```python
from build123d import *

# Parameters (mm, degrees)
F0_R     = 4.25
F1_DEPTH = 55
F2_R     = 4.25
F2_R_2   = 0.35
F3_DEPTH = 3
F4_R     = 4.25
F5_DEPTH = 3
F7_DEPTH = 25


with BuildPart() as f1:
    # F0 (on Top) → F1 (new body)
    with BuildSketch(Plane.XY):
        Circle(F0_R)
        with BuildLine():
            ThreePointArc((0.4014783638, -0.4458868953), (0, -0.6), (-0.4014783638, -0.4458868953))
            Line((-0.4014783638, -0.4458868953), (-1.7825704497, -3.1564327321))
            ThreePointArc((-1.7825704497, -3.1564327321), (-2.1167558909, -2.9427826114), (-2.4255984481, -2.6938999924))
            ThreePointArc((-2.4255984481, -2.6938999924), (-3.1393420887, -1.8125), (-3.5457850527, -0.7536798792))
            ThreePointArc((-3.5457850527, -0.7536798792), (-3.6069024448, -0.3617730694), (-3.6248361561, 0.0344650726))
            Line((-3.6248361561, 0.0344650726), (-0.5868885604, -0.1247470145))
            ThreePointArc((-0.5868885604, -0.1247470145), (-0.5196152423, 0.3), (-0.1854101966, 0.5706339098))
            Line((-0.1854101966, 0.5706339098), (-1.8422657065, 3.1219676595))
            ThreePointArc((-1.8422657065, 3.1219676595), (0, 3.625), (1.8422657065, 3.1219676595))
            Line((1.8422657065, 3.1219676595), (0.1854101966, 0.5706339098))
            ThreePointArc((0.1854101966, 0.5706339098), (0.5196152423, 0.3), (0.5868885604, -0.1247470145))
            Line((0.5868885604, -0.1247470145), (3.6248361561, 0.0344650726))
            ThreePointArc((3.6248361561, 0.0344650726), (3.1393420887, -1.8125), (1.7825704497, -3.1564327321))
            Line((1.7825704497, -3.1564327321), (0.4014783638, -0.4458868953))
        make_face(mode=Mode.SUBTRACT)
    extrude(amount=F1_DEPTH)

    # F2 (on face) → F3 (join)
    with BuildSketch(Plane.XY.offset(55)):
        Circle(F2_R)
        Circle(F2_R_2, mode=Mode.SUBTRACT)
    extrude(amount=F3_DEPTH)

    # F4 (on face) → F5 (join)
    with BuildSketch(Plane.XY.offset(58)):
        Circle(F4_R)
    extrude(amount=F5_DEPTH)

    # F6 (on face) → F7 (join)
    with BuildSketch(Plane.XY.offset(61)):
        with BuildLine():
            ThreePointArc((-2.843805077, -3.1583655083), (-3.6806079661, -2.125), (-4.1571273031, -0.883624686))
            Line((-4.1571273031, -0.883624686), (-5.4765591727, -1.1640785875))
            ThreePointArc((-5.4765591727, -1.1640785875), (-4.8487972217, -2.7994543812), (-3.7464012151, -4.1608000751))
            Line((-3.7464012151, -4.1608000751), (-2.843805077, -3.1583655083))
        make_face()
        with BuildLine():
            ThreePointArc((-1.3133222261, 4.0419901943), (0, 4.25), (1.3133222261, 4.0419901943))
            Line((1.3133222261, 4.0419901943), (1.7301579575, 5.3248786626))
            ThreePointArc((1.7301579575, 5.3248786626), (0, 5.5989087624), (-1.7301579575, 5.3248786626))
            Line((-1.7301579575, 5.3248786626), (-1.3133222261, 4.0419901943))
        make_face()
        with BuildLine():
            ThreePointArc((4.1571273031, -0.883624686), (3.6806079661, -2.125), (2.843805077, -3.1583655083))
            Line((2.843805077, -3.1583655083), (3.7464012151, -4.1608000751))
            ThreePointArc((3.7464012151, -4.1608000751), (4.8487972217, -2.7994543812), (5.4765591727, -1.1640785875))
            Line((5.4765591727, -1.1640785875), (4.1571273031, -0.883624686))
        make_face()
    extrude(amount=-F7_DEPTH)


solid = f1.part
```
Read the model definition and answer for the solid it produces. Units are mm, in the model's axes. A direction names the side the tool comes from. Coordinates: 2 decimals unless noted, no trailing zeros. Loops run counter-clockwise (first coordinate to the right, second up) from the corner with the lowest first, then second, coordinate; pieces in that order, holes last.
(1) The part is cut by section A-A (z = 14.5). Determine the outline of the cut face in (x, y) (3 decimals).
Solution:
outline: circle Ø8.5 at (0, 0); hole (-3.625, 0.034) arc R3.625 ccw to (-1.783, -3.156) - (-0.401, -0.446) arc R0.6 ccw to (0.401, -0.446) - (1.783, -3.156) arc R3.625 ccw to (3.625, 0.034) - (0.587, -0.125) arc R0.6 ccw to (0.185, 0.571) - (1.842, 3.122) arc R3.625 ccw to (-1.842, 3.122) - (-0.185, 0.571) arc R0.6 ccw to (-0.587, -0.125) - close
(2) The part is cut by section B-B (z = 39). Determine the outline of the cut face in (x, y) (3 decimals).
Solution:
outline: (-5.477, -1.164) arc R5.599 ccw to (-3.746, -4.161) - (-2.844, -3.158) arc R4.25 ccw to (2.844, -3.158) - (3.746, -4.161) arc R5.599 ccw to (5.477, -1.164) - (4.157, -0.884) arc R4.25 ccw to (1.313, 4.042) - (1.73, 5.325) arc R5.599 ccw to (-1.73, 5.325) - (-1.313, 4.042) arc R4.25 ccw to (-4.157, -0.884) - close; hole (-3.625, 0.034) arc R3.625 ccw to (-1.783, -3.156) - (-0.401, -0.446) arc R0.6 ccw to (0.401, -0.446) - (1.783, -3.156) arc R3.625 ccw to (3.625, 0.034) - (0.587, -0.125) arc R0.6 ccw to (0.185, 0.571) - (1.842, 3.122) arc R3.625 ccw to (-1.842, 3.122) - (-0.185, 0.571) arc R0.6 ccw to (-0.587, -0.125) - close
(3) The mould has two halves that part along Y. Classify faces 4 (the face through (-4, -2, 36)), 5 (the face through (3.289, -3.653, 48.675)), 6 (the face through (-1.002, 1.828, 27.115)): released by +Y, released by -Y, zero draft, split by the parting line, or undercut.
Solution:
face 4: zero draft
face 5: released by -Y
face 6: undercut
(4) Consider line 1 along Y through (x, z) = (0, 56.3); line 2 along X through (y, z) = (-3.25, 38); line 3 along Y through (x, z) = (-1.5, 33). Determine where each line is inside the solid, lowest interval first.
Solution:
line 1: y = -4.25 to -0.35, 0.35 to 5.6
line 2: x = -4.56 to -2.93, -2.74 to 2.74, 2.93 to 4.56
line 3: y = -3.98 to -2.6, -0.08 to 2.59, 3.3 to 3.98
(5) Flat-ended cylindrical pins translate along their axes: pin 1 Ø1 at (y, z) = (0.5, 22) entering from -X; pin 2 Ø3 at (x, y) = (-4, -2.5) entering from -Z; pin 3 Ø1 at (x, z) = (4, 17.5) entering from -Y; pin 4 Ø2 at (x, y) = (4.5, -3) entering from -Z. Find the tip coordinate at first contact, or state that the pin passes through.
Solution:
pin 1: stops at x = -4.25
pin 2: stops at z = 0
pin 3: stops at y = -2.41
pin 4: stops at z = 36
(6) A tool of negligible diameter and unlimited length cuts with its end or side. For faces 1 (the face through (1.519, 4.674, 48.675)), 2 (the face through (1.1, -1.82, 27.12)), 3 (the face through (4, -2, 36)), from which of +Z, -Z, +X, -X, +Y, -Y can it reach the whole face along a straight path? Write none if from no direction.
Solution:
face 1: +Z, -Z, +X
face 2: -Z
face 3: -Z, +X, -Y
